```python
from build123d import *

# Parameters (mm, degrees)
EXTRUDE_1_DEPTH = 2.6
SKETCH_2_R      = 3.5
SKETCH_2_R_2    = 2.95
EXTRUDE_2_DEPTH = 2.5


with BuildPart() as part:
    # ｽｹｯﾁ1 → ﾎﾞｽ - 押し出し1 (new body)
    with BuildSketch(Plane.XY):
        Polygon((11.29842378, 0.078571429), (20.79842378, 0.078571429), (20.79842378, 9.578571429), (27.79842378, 9.578571429), (27.79842378, 0.078571429), (37.29842378, 0.078571429), (37.29842378, -6.921428571), (27.79842378, -6.921428571), (27.79842378, -16.421428571), (20.79842378, -16.421428571), (20.79842378, -6.921428571), (11.29842378, -6.921428571), align=None)
    extrude(amount=EXTRUDE_1_DEPTH)

    # ｽｹｯﾁ2 → ﾎﾞｽ - 押し出し2 (add)
    with BuildSketch(Plane.XY.offset(2.6)):
        with Locations((24.29842378, -3.421428571)):
            Circle(SKETCH_2_R)
        with Locations((24.29842378, -3.421428571)):
            Circle(SKETCH_2_R_2, mode=Mode.SUBTRACT)
    extrude(amount=EXTRUDE_2_DEPTH)


solid = part.part
```
Here's how the part is built. I have some questions about the finished solid (model axes, mm). A direction names the side the tool comes from. Give positions to 0.01 mm unless a question says otherwise; leave off trailing zeros. Order: outer loops, then holes, each group sorted by start corner. A loop starts at its lowest first (then second) coordinate and runs counter-clockwise, first axis right, second up. Notation, with made-up numbers: (22, 55) - (78, 55) arc R34 ccw to (78, 91) - close; hole circle Ø6 at (-18.75, 61.5). An arc over 180 degrees is marked (long way). Answer as a JSON object with one key per item and string values. Group by question number.
Item 1: If we section it at A-A on z = 1.7: Please give me the cut outline in (x, y).
Item 2: If we section it at B-B on x = 23.25: Please give me the cut outline in (y, z), and give its area (3 significant figures).
Item 3: If we mould it in two halves opening along X, with no side actions, what happens to faces 6 (the flat face through (24, -3, 2.6)), 7 (the flat face through (20.798, 5, 1)), 8 (the flat face through (27.798, 5, 1)), 9 (the flat face through (21, -4, 5.1))? For each: pulls with the +X half, pulls with the -X half, needs draft (parallel to the pull), parting line crosses it, or undercut.
Item 4: Please list where these lines run through material, in increasing order: probe 1 along X at (y, z) = (6, 2.2); probe 2 along Y at (x, z) = (32.5, 0.65); probe 3 along Z at (x, y) = (25.5, 2.5).
Item 5: If we section it at C-C on y = 4.75: Please give me the cut outline in (x, z).
Item 6: Which directions (+Z, -Z, +X, -X, +Y, -Y) give clear straight access to the entire face, cutting with the end or side of a thin tool? Please do faces 1 (the flat face through (16, -6.921, 1)), 2 (the flat face through (16, 0.079, 1)), 3 (the cylindrical face through (20.8, -3.3, 3.8)), 4 (the flat face through (32, 0.079, 1)), 5 (the flat face through (33, -6.921, 1)).
Item 7: For P1, Ø0.8, axis at x = 13.5, z = 1, coming from the -Y side; P2, Ø3, axis at x = 25.5, y = -9, coming from the -Z side; P3, Ø2, axis at y = -5.5, z = 4, coming from the +X side; P4, Ø3, axis at y = 6.5, z = 2, coming from the +X side, each with a flat end and sliding along its axis, tell me the tip position at first contact or that it passes through.
Item 8: If we section it at D-D on z = 4.7: Please give me the cut outline in (x, y).
Result set:
{
 "1": {"outline": "(11.3, -6.92) - (20.8, -6.92) - (20.8, -16.42) - (27.8, -16.42) - (27.8, -6.92) - (37.3, -6.92) - (37.3, 0.08) - (27.8, 0.08) - (27.8, 9.58) - (20.8, 9.58) - (20.8, 0.08) - (11.3, 0.08) - close"},
 "2": {"outline": "(-16.42, 0) - (9.58, 0) - (9.58, 2.6) - (-0.08, 2.6) - (-0.08, 5.1) - (-0.66, 5.1) - (-0.66, 2.6) - (-6.18, 2.6) - (-6.18, 5.1) - (-6.76, 5.1) - (-6.76, 2.6) - (-16.42, 2.6) - close", "area": "70.5 mm²"},
 "3": {"face 6": "undercut", "face 7": "pulls with the -X half", "face 8": "pulls with the +X half", "face 9": "needs draft"},
 "4": {"probe 1": "20.8 to 27.8", "probe 2": "-6.92 to 0.08", "probe 3": "0 to 2.6"},
 "5": {"outline": "(20.8, 0) - (27.8, 0) - (27.8, 2.6) - (20.8, 2.6) - close"},
 "6": {"face 1": "+Z, -Z, -X, -Y", "face 2": "+Z, -Z, -X, +Y", "face 3": "+Z", "face 4": "+Z, -Z, +X, +Y", "face 5": "+Z, -Z, +X, -Y"},
 "7": {"P1": "y = -6.92", "P2": "z = 0", "P3": "x = 27.63", "P4": "x = 27.8"},
 "8": {"outline": "circle Ø7 at (24.3, -3.42); hole circle Ø5.9 at (24.3, -3.42)"}
}
